from build123d import *

# Parameters (mm, degrees)
EXTRUDE2_DEPTH = 4.445


with BuildPart() as part:
    # Sketch1 → Extrude2 (new body)
    with BuildSketch(Plane(origin=(0, 0, 0), x_dir=(1, 0, 0), z_dir=(0, 1, 0))):
        with BuildLine():
            Line((0, 0), (70.128669853, 0))
            ThreePointArc((70.128669853, 0), (91.447571558, 21.318901704), (70.128669853, 42.637803409))
            Line((70.128669853, 42.637803409), (56.809824029, 42.637803409))
            ThreePointArc((56.809824029, 42.637803409), (54.625693022, 43.025247602), (52.708090795, 44.140300497))
            Line((52.708090795, 44.140300497), (39.921942966, 54.95934866))
            ThreePointArc((39.921942966, 54.95934866), (38.004340739, 56.074401554), (35.820209733, 56.461845748))
            Line((35.820209733, 56.461845748), (0, 56.461845748))
            Line((0, 56.461845748), (0, 0))
        make_face()
    extrude(amount=-EXTRUDE2_DEPTH)


solid = part.part
Can you work these out from the model? Positions are in its coordinate system, mm. A direction names the side the tool comes from. Give positions to 0.01 mm unless a question says otherwise; leave off trailing zeros. Loops run counter-clockwise (first coordinate to the right, second up) from the corner with the lowest first, then second, coordinate; pieces in that order, holes last. Notation, with made-up numbers: (17.25, 86) - (44.25, 86) arc R33 cw to (44.25, 121) - close; hole circle Ø9 at (14.25, 44.25). An arc over 180 degrees is marked (long way). One line per item, written item: value.
(1) I need wall thicknesses on line 1 along Z through (x, y) = (57.5, -2.6); line 2 along X through (y, z) = (-2.5, -21.5); line 3 along X through (y, z) = (-2.1, -6). Which ranges of each line are inside material? Lowest first, please.
Verdict:
line 1: -42.64 to 0
line 2: 0 to 91.45
line 3: 0 to 84.96
(2) I'm going to push a flat-ended pin straight in: pin 1 (1.5 mm diameter, centred on x = 39, y = -2.5, fed in from -Z). Where does the tip first touch, or does it pass through?
Verdict:
pin 1: z = -55.98
(3) If we section it at B-B, the plane z = -38: List the corners of the cut face in (x, y) for me (3 decimals).
Verdict:
outline: (0, -4.445) - (83.404, -4.445) - (83.404, 0) - (0, 0) - close
(4) If we section it at C-C, the plane x = 66.5: List the corners of the cut face in (y, z) for me (3 decimals), plus the area to 3 significant figures.
Verdict:
outline: (-4.445, -42.638) - (0, -42.638) - (0, 0) - (-4.445, 0) - close
area: 190 mm^2
(5) If we section it at A-A, the plane y = -3: List the corners of the cut face in (x, z) for me, plus the area to 3 significant figures.
Verdict:
outline: (0, -56.46) - (35.82, -56.46) arc R6.35 ccw to (39.92, -54.96) - (52.71, -44.14) arc R6.35 cw to (56.81, -42.64) - (70.13, -42.64) arc R21.32 ccw to (70.13, 0) - (0, 0) - close
area: 4,340 mm^2
(6) On a 3-axis mill with a long thin cutter (end or side, diameter ignored), from which of +Z, -Z, +X, -X, +Y, -Y can I reach the whole of each face in a straight line? I mean faces 1 (the face through (64, -2, -42.638)), 2 (the face through (45, -4.445, -29)). Say none if no direction works.
Verdict:
face 1: -Z, +X, +Y, -Y
face 2: +Z, -Z, +X, -X, -Y
